Design review of the part built by this model. Coordinates are the model's own, in mm. A direction names the side the tool comes from. Coordinates: 2 decimals unless noted, no trailing zeros. Loops run counter-clockwise (first coordinate to the right, second up) from the corner with the lowest first, then second, coordinate; pieces in that order, holes last. Notation, with made-up numbers: (-30.5, 28) - (3.5, 28) arc R28 cw to (3.5, 64) - close; hole circle Ø11 at (60, 28.5). An arc over 180 degrees is marked (long way). Answer in a Markdown table with one row per item. Add a question column.
(1) We need section C-C, the plane x = 42. Write out the cut boundary in (y, z), plus the area to 3 significant figures.
(2) For faces 4 (the face through (-66, 65, -5)), 5 (the face through (-66, 37, -60)), 6 (the face through (-52, 32, -2)), list the 3-axis set-ups (+Z, -Z, +X, -X, +Y, -Y) from which the entire face can be reached by the end or side of a thin tool; tool diameter is ignored.
(3) We need section B-B, the plane z = -98.5. Write out the cut boundary in (x, y), plus the area to 3 significant figures.
(4) We need section D-D, the plane y = 33. Give the number of separate pieces and of enclosed holes in the cut face, plus the area to 3 significant figures.
(5) The part is to be moulded in two halves that separate along X. For faces 1 (the face through (-3, 65, -8)), 2 (the face through (-71, 32, -179)), 3 (the face through (34, 10, -100)), say which applies: released by +X, released by -X, zero draft, split by the parting line, or undercut.
(6) To check wall thickness, follow L1, parallel to Z at x = -35, y = 8; L2, parallel to X at y = 13, z = -140.5; L3, parallel to X at y = 7.05, z = -162.5. State the ranges of each line that lie inside material, in increasing order. Write a range as [from, to].
(7) Clearance check with flat-ended pins moving along their axes: pin 1 (4.5 mm diameter, centred on x = -15, y = 47.5, fed in from +Z); pin 2 (10 mm diameter, centred on x = 143, y = 18, fed in from +Z); pin 3 (12 mm diameter, centred on x = 97.5, z = -71, fed in from +Y); pin 4 (8 mm diameter, centred on y = 28, z = -154.5, fed in from -X). State where each tip first meets the part, or that it passes through.
(8) We need section A-A, the plane x = -35.5. Write out the cut boundary in (y, z), plus the area to 3 significant figures.
from build123d import *
from OCP.BRepFilletAPI import BRepFilletAPI_MakeChamfer

# Parameters (mm, degrees)
BOARDBASE_DEPTH     = 10
SKETCH1_6_W         = 200
SKETCH1_6_H         = 200
SKETCH1_6_W_2       = 61
SKETCH1_6_H_2       = 61
PIECEHOLDERS_DEPTH  = 15
PIECESLIDEAID_SIZE  = 1
PIECESLIDEAID_SIZE2 = 1.732050808
BOSS_EXTRUDE3_DEPTH = 65
SKETCH4_R           = 18.5
CUT_EXTRUDE1_DEPTH  = 5


with BuildPart() as part:
    # Sketch1 → BoardBase (new body)
    with BuildSketch(Plane(origin=(0, 0, 0), x_dir=(1, 0, 0), z_dir=(0, 1, 0))):
        Polygon((0, 2), (0, 0), (200, 0), (200, 200), (0, 200), (0, 198), (-71, 198), (-71, 127), (0, 127), (0, 73), (-71, 73), (-71, 2), align=None)
    extrude(amount=BOARDBASE_DEPTH)

    # Sketch1<6> → PieceHolders (add)
    with BuildSketch(Plane(origin=(0, 0, 0), x_dir=(1, 0, 0), z_dir=(0, 1, 0))):
        with Locations((100, 100)):
            Rectangle(SKETCH1_6_W, SKETCH1_6_H)
        with Locations((34.75, 165.25)):
            Rectangle(SKETCH1_6_W_2, SKETCH1_6_H_2, mode=Mode.SUBTRACT)
        with Locations((100, 165.25)):
            Rectangle(SKETCH1_6_W_2, SKETCH1_6_H_2, mode=Mode.SUBTRACT)
        with Locations((165.25, 165.25)):
            Rectangle(SKETCH1_6_W_2, SKETCH1_6_H_2, mode=Mode.SUBTRACT)
        with Locations((34.75, 100)):
            Rectangle(SKETCH1_6_W_2, SKETCH1_6_H_2, mode=Mode.SUBTRACT)
        with Locations((100, 100)):
            Rectangle(SKETCH1_6_W_2, SKETCH1_6_H_2, mode=Mode.SUBTRACT)
        with Locations((165.25, 100)):
            Rectangle(SKETCH1_6_W_2, SKETCH1_6_H_2, mode=Mode.SUBTRACT)
        with Locations((34.75, 34.75)):
            Rectangle(SKETCH1_6_W_2, SKETCH1_6_H_2, mode=Mode.SUBTRACT)
        with Locations((100, 34.75)):
            Rectangle(SKETCH1_6_W_2, SKETCH1_6_H_2, mode=Mode.SUBTRACT)
        with Locations((165.25, 34.75)):
            Rectangle(SKETCH1_6_W_2, SKETCH1_6_H_2, mode=Mode.SUBTRACT)
    extrude(amount=PIECEHOLDERS_DEPTH)

    # PieceSlideAid: one chamfer whose edges measure the first distance from different faces: ONE call of the kernel's chamfer builder (chamfer() names one face for all edges)
    pieceslideaid_edges_1 = [part.edges().sort_by_distance(p)[0] for p in [
        (165.25, 15, -4.25),
        (100, 15, -4.25),
        (165.25, 15, -69.5),
        (165.25, 15, -134.75),
        (100, 15, -134.75),
        (69.5, 15, -34.75),
        (134.75, 15, -100),
        (134.75, 15, -165.25),
        (69.5, 15, -165.25),
        (134.75, 15, -34.75),
        (100, 15, -195.75),
        (130.5, 15, -165.25),
        (165.25, 15, -195.75),
        (195.75, 15, -165.25),
        (165.25, 15, -130.5),
        (195.75, 15, -100),
        (100, 15, -65.25),
        (130.5, 15, -34.75),
        (165.25, 15, -65.25),
        (195.75, 15, -34.75),
    ]]
    pieceslideaid_side_1 = [part.faces().sort_by_distance(p)[0] for p in [
        (100, 15, -2.828427125),
    ]]
    pieceslideaid_edges_2 = [part.edges().sort_by_distance(p)[0] for p in [
        (34.75, 15, -4.25),
    ]]
    pieceslideaid_side_2 = [part.faces().sort_by_distance(p)[0] for p in [
        (34.75, 12.5, -4.25),
    ]]
    pieceslideaid_edges_3 = [part.edges().sort_by_distance(p)[0] for p in [
        (100, 15, -69.5),
    ]]
    pieceslideaid_side_3 = [part.faces().sort_by_distance(p)[0] for p in [
        (100, 12.5, -69.5),
    ]]
    pieceslideaid_edges_4 = [part.edges().sort_by_distance(p)[0] for p in [
        (34.75, 15, -69.5),
    ]]
    pieceslideaid_side_4 = [part.faces().sort_by_distance(p)[0] for p in [
        (34.75, 12.5, -69.5),
    ]]
    pieceslideaid_edges_5 = [part.edges().sort_by_distance(p)[0] for p in [
        (34.75, 15, -134.75),
    ]]
    pieceslideaid_side_5 = [part.faces().sort_by_distance(p)[0] for p in [
        (34.75, 12.5, -134.75),
    ]]
    pieceslideaid_edges_6 = [part.edges().sort_by_distance(p)[0] for p in [
        (4.25, 15, -34.75),
    ]]
    pieceslideaid_side_6 = [part.faces().sort_by_distance(p)[0] for p in [
        (4.25, 12.5, -34.75),
    ]]
    pieceslideaid_edges_7 = [part.edges().sort_by_distance(p)[0] for p in [
        (69.5, 15, -100),
    ]]
    pieceslideaid_side_7 = [part.faces().sort_by_distance(p)[0] for p in [
        (69.5, 12.5, -100),
    ]]
    pieceslideaid_edges_8 = [part.edges().sort_by_distance(p)[0] for p in [
        (4.25, 15, -100),
    ]]
    pieceslideaid_side_8 = [part.faces().sort_by_distance(p)[0] for p in [
        (4.25, 12.5, -100),
    ]]
    pieceslideaid_edges_9 = [part.edges().sort_by_distance(p)[0] for p in [
        (4.25, 15, -165.25),
    ]]
    pieceslideaid_side_9 = [part.faces().sort_by_distance(p)[0] for p in [
        (4.25, 12.5, -165.25),
    ]]
    pieceslideaid_edges_10 = [part.edges().sort_by_distance(p)[0] for p in [
        (34.75, 15, -195.75),
    ]]
    pieceslideaid_side_10 = [part.faces().sort_by_distance(p)[0] for p in [
        (34.75, 12.5, -195.75),
    ]]
    pieceslideaid_edges_11 = [part.edges().sort_by_distance(p)[0] for p in [
        (65.25, 15, -165.25),
    ]]
    pieceslideaid_side_11 = [part.faces().sort_by_distance(p)[0] for p in [
        (65.25, 12.5, -165.25),
    ]]
    pieceslideaid_edges_12 = [part.edges().sort_by_distance(p)[0] for p in [
        (34.75, 15, -130.5),
    ]]
    pieceslideaid_side_12 = [part.faces().sort_by_distance(p)[0] for p in [
        (34.75, 12.5, -130.5),
    ]]
    pieceslideaid_edges_13 = [part.edges().sort_by_distance(p)[0] for p in [
        (65.25, 15, -100),
    ]]
    pieceslideaid_side_13 = [part.faces().sort_by_distance(p)[0] for p in [
        (65.25, 12.5, -100),
    ]]
    pieceslideaid_edges_14 = [part.edges().sort_by_distance(p)[0] for p in [
        (100, 15, -130.5),
    ]]
    pieceslideaid_side_14 = [part.faces().sort_by_distance(p)[0] for p in [
        (100, 12.5, -130.5),
    ]]
    pieceslideaid_edges_15 = [part.edges().sort_by_distance(p)[0] for p in [
        (130.5, 15, -100),
    ]]
    pieceslideaid_side_15 = [part.faces().sort_by_distance(p)[0] for p in [
        (130.5, 12.5, -100),
    ]]
    pieceslideaid_edges_16 = [part.edges().sort_by_distance(p)[0] for p in [
        (34.75, 15, -65.25),
    ]]
    pieceslideaid_side_16 = [part.faces().sort_by_distance(p)[0] for p in [
        (34.75, 12.5, -65.25),
    ]]
    pieceslideaid_edges_17 = [part.edges().sort_by_distance(p)[0] for p in [
        (65.25, 15, -34.75),
    ]]
    pieceslideaid_side_17 = [part.faces().sort_by_distance(p)[0] for p in [
        (65.25, 12.5, -34.75),
    ]]
    pieceslideaid = BRepFilletAPI_MakeChamfer(part.part.solid().wrapped)
    for e in pieceslideaid_edges_1:
        pieceslideaid.Add(PIECESLIDEAID_SIZE, PIECESLIDEAID_SIZE2, e.wrapped, pieceslideaid_side_1[0].wrapped)  # the first distance lies on this face
    for e in pieceslideaid_edges_2:
        pieceslideaid.Add(PIECESLIDEAID_SIZE, PIECESLIDEAID_SIZE2, e.wrapped, pieceslideaid_side_2[0].wrapped)  # the first distance lies on this face
    for e in pieceslideaid_edges_3:
        pieceslideaid.Add(PIECESLIDEAID_SIZE, PIECESLIDEAID_SIZE2, e.wrapped, pieceslideaid_side_3[0].wrapped)  # the first distance lies on this face
    for e in pieceslideaid_edges_4:
        pieceslideaid.Add(PIECESLIDEAID_SIZE, PIECESLIDEAID_SIZE2, e.wrapped, pieceslideaid_side_4[0].wrapped)  # the first distance lies on this face
    for e in pieceslideaid_edges_5:
        pieceslideaid.Add(PIECESLIDEAID_SIZE, PIECESLIDEAID_SIZE2, e.wrapped, pieceslideaid_side_5[0].wrapped)  # the first distance lies on this face
    for e in pieceslideaid_edges_6:
        pieceslideaid.Add(PIECESLIDEAID_SIZE, PIECESLIDEAID_SIZE2, e.wrapped, pieceslideaid_side_6[0].wrapped)  # the first distance lies on this face
    for e in pieceslideaid_edges_7:
        pieceslideaid.Add(PIECESLIDEAID_SIZE, PIECESLIDEAID_SIZE2, e.wrapped, pieceslideaid_side_7[0].wrapped)  # the first distance lies on this face
    for e in pieceslideaid_edges_8:
        pieceslideaid.Add(PIECESLIDEAID_SIZE, PIECESLIDEAID_SIZE2, e.wrapped, pieceslideaid_side_8[0].wrapped)  # the first distance lies on this face
    for e in pieceslideaid_edges_9:
        pieceslideaid.Add(PIECESLIDEAID_SIZE, PIECESLIDEAID_SIZE2, e.wrapped, pieceslideaid_side_9[0].wrapped)  # the first distance lies on this face
    for e in pieceslideaid_edges_10:
        pieceslideaid.Add(PIECESLIDEAID_SIZE, PIECESLIDEAID_SIZE2, e.wrapped, pieceslideaid_side_10[0].wrapped)  # the first distance lies on this face
    for e in pieceslideaid_edges_11:
        pieceslideaid.Add(PIECESLIDEAID_SIZE, PIECESLIDEAID_SIZE2, e.wrapped, pieceslideaid_side_11[0].wrapped)  # the first distance lies on this face
    for e in pieceslideaid_edges_12:
        pieceslideaid.Add(PIECESLIDEAID_SIZE, PIECESLIDEAID_SIZE2, e.wrapped, pieceslideaid_side_12[0].wrapped)  # the first distance lies on this face
    for e in pieceslideaid_edges_13:
        pieceslideaid.Add(PIECESLIDEAID_SIZE, PIECESLIDEAID_SIZE2, e.wrapped, pieceslideaid_side_13[0].wrapped)  # the first distance lies on this face
    for e in pieceslideaid_edges_14:
        pieceslideaid.Add(PIECESLIDEAID_SIZE, PIECESLIDEAID_SIZE2, e.wrapped, pieceslideaid_side_14[0].wrapped)  # the first distance lies on this face
    for e in pieceslideaid_edges_15:
        pieceslideaid.Add(PIECESLIDEAID_SIZE, PIECESLIDEAID_SIZE2, e.wrapped, pieceslideaid_side_15[0].wrapped)  # the first distance lies on this face
    for e in pieceslideaid_edges_16:
        pieceslideaid.Add(PIECESLIDEAID_SIZE, PIECESLIDEAID_SIZE2, e.wrapped, pieceslideaid_side_16[0].wrapped)  # the first distance lies on this face
    for e in pieceslideaid_edges_17:
        pieceslideaid.Add(PIECESLIDEAID_SIZE, PIECESLIDEAID_SIZE2, e.wrapped, pieceslideaid_side_17[0].wrapped)  # the first distance lies on this face
    add(Compound.cast(pieceslideaid.Shape()), mode=Mode.REPLACE)

    # Sketch1<8> → Boss-Extrude3 (add)
    with BuildSketch(Plane(origin=(0, 0, 0), x_dir=(1, 0, 0), z_dir=(0, 1, 0))):
        Polygon((-71, 127), (-51, 127), (-51, 132), (-66, 132), (-66, 147), (-71, 147), align=None)
        Polygon((-51, 193), (-51, 198), (-71, 198), (-71, 178), (-66, 178), (-66, 193), align=None)
        Polygon((0, 178), (0, 198), (-20, 198), (-20, 193), (-5, 193), (-5, 178), align=None)
        Polygon((-20, 127), (0, 127), (0, 147), (-5, 147), (-5, 132), (-20, 132), align=None)
        Polygon((-51, 68), (-51, 73), (-71, 73), (-71, 53), (-66, 53), (-66, 68), align=None)
        Polygon((-71, 2), (-51, 2), (-51, 7), (-66, 7), (-66, 22), (-71, 22), align=None)
        Polygon((-20, 2), (0, 2), (0, 22), (-5, 22), (-5, 7), (-20, 7), align=None)
        Polygon((-5, 53), (0, 53), (0, 73), (-20, 73), (-20, 68), (-5, 68), align=None)
    extrude(amount=BOSS_EXTRUDE3_DEPTH)

    # Sketch4 → Cut-Extrude1 (cut)
    with BuildSketch(Plane(origin=(0, 10, 0), x_dir=(1, 0, 0), z_dir=(0, 1, 0))):
        with Locations(Location((-35.5, 37.5, 0), (0, 0, 270))):
            Circle(SKETCH4_R)
        with Locations(Location((-35.5, 162.5, 0), (0, 0, 270))):
            Circle(SKETCH4_R)
    extrude(amount=-CUT_EXTRUDE1_DEPTH, mode=Mode.SUBTRACT)


solid = part.part
Responses:
| question | item | result |
|---|---|---|
| 1 | outline | (0, -200) - (15, -200) - (15, -197.48) - (14, -195.75) - (10, -195.75) - (10, -134.75) - (14, -134.75) - (15, -133.02) - (15, -132.23) - (14, -130.5) - (10, -130.5) - (10, -69.5) - (14, -69.5) - (15, -67.77) - (15, -66.98) - (14, -65.25) - (10, -65.25) - (10, -4.25) - (14, -4.25) - (15, -2.52) - (15, 0) - (0, 0) - close |
| 1 | area | 2,080 mm2 |
| 2 | face 4 | +Z, -Z, +X, -X, +Y |
| 2 | face 5 | +Y |
| 2 | face 6 | +Z, -X, +Y, -Y |
| 3 | outline | (0, 0) - (200, 0) - (200, 15) - (196.75, 15) - (195.75, 13.27) - (195.75, 10) - (134.75, 10) - (134.75, 13.27) - (133.75, 15) - (132.23, 15) - (130.5, 14) - (130.5, 10) - (69.5, 10) - (69.5, 14) - (67.77, 15) - (66.98, 15) - (65.25, 14) - (65.25, 10) - (4.25, 10) - (4.25, 14) - (2.52, 15) - (0, 15) - close |
| 3 | area | 2,080 mm2 |
| 4 | separate pieces | 8 |
| 4 | enclosed holes | 0 |
| 4 | area | 1,400 mm2 |
| 5 | face 1 | zero draft |
| 5 | face 2 | released by -X |
| 5 | face 3 | undercut |
| 6 | L1 | z = [-198, -180.99], [-144.01, -127], [-73, -55.99], [-19.01, -2] |
| 6 | L2 | x = [-71, -66], [-5, 4.25], [65.25, 69.5], [130.5, 134.75], [195.75, 200] |
| 6 | L3 | x = [-71, -54], [-17, 200] |
| 7 | pin 1 | stops at z = -2 |
| 7 | pin 2 | stops at z = 0 |
| 7 | pin 3 | stops at y = 15 |
| 7 | pin 4 | passes through |
| 8 | outline | (0, -198) - (10, -198) - (10, -181) - (5, -181) - (5, -144) - (10, -144) - (10, -127) - (0, -127) - close; (0, -73) - (10, -73) - (10, -56) - (5, -56) - (5, -19) - (10, -19) - (10, -2) - (0, -2) - close |
| 8 | area | 1,050 mm2 |
